Source: CAD feature listing. Evaluate the final solid. Frame: model axes, mm. Coordinates: 2 decimals unless noted, no trailing zeros. Order: outer loops, then holes, each group sorted by start corner. A loop starts at its lowest first (then second) coordinate and runs counter-clockwise, first axis right, second up. Notation, with made-up numbers: (50, -2) - (89, -2) arc R30 cw to (89, 30) - close; hole circle Ø11 at (43, 57.25). An arc over 180 degrees is marked (long way). One line per question, with ' | ' between items. Start each with the question number.
(1) Contact query for flat-ended pins moving along their axis: P1, Ø8, axis at x = -2.5, y = -0.5, coming from the +Z side; P2, Ø1.9, axis at x = 0, z = -163, coming from the -Y side; P3, Ø4, axis at x = 0, z = -163, coming from the +Y side. Output: stop coordinate, or through.
(2) Line query: line 1 along Z through (x, y) = (0, 8.9); line 2 along Y through (x, z) = (1.25, -27.5); line 3 along Z through (x, y) = (5.5, 7). Output: solid intervals per line, ascending.
(3) Section A-A (z = -77.5). Return the cut outline in (x, y).
(4) Section B-B (y = 0). Return the cut outline in (x, z), then the cut area to 3 significant figures.
(5) Section C-C (z = -163). Return the cut outline in (x, y).
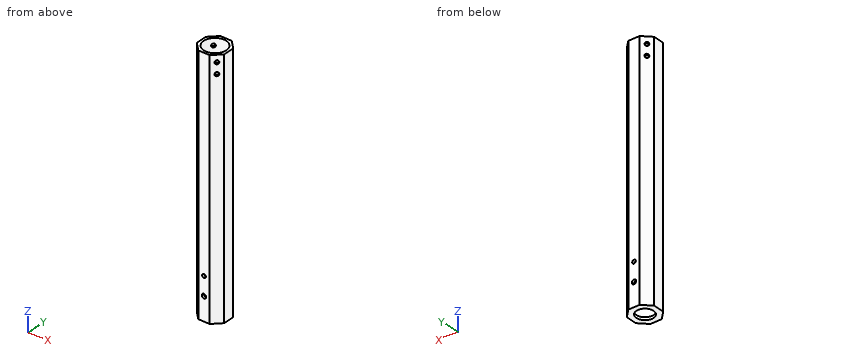
from build123d import *

# Parameters (mm, degrees)
SKETCH1_R               = 8.25
BOSS_EXTRUDE1_DEPTH     = 178
BOSS_EXTRUDE2_DEPTH     = 2
CUT_EXTRUDE1_DEPTH      = 181.554700853
CUT_EXTRUDE1_DEPTH_BACK = 181.554700853
SKETCH4_R               = 1.35
SKETCH4_R_2             = 1.6
SKETCH6_R               = 1.4
CUT_EXTRUDE2_DEPTH      = 182.611791236
CIRPATTERN1_COUNT       = 2
CIRPATTERN1_ANGLE       = 270
SKETCH7_R               = 6.269832862
CUT_EXTRUDE3_DEPTH      = 181.554700958


with BuildPart() as part:
    # Sketch1 → Boss-Extrude1 (new body)
    with BuildSketch(Plane.XY):
        Polygon((10, 4.142135624), (4.142135624, 10), (-4.142135624, 10), (-10, 4.142135624), (-10, -4.142135624), (-4.142135624, -10), (4.142135624, -10), (10, -4.142135624), align=None)
        Circle(SKETCH1_R, mode=Mode.SUBTRACT)
    extrude(amount=-BOSS_EXTRUDE1_DEPTH)

    # Sketch2 → Boss-Extrude2 (add)
    with BuildSketch(Plane(origin=(0, 0, -178), x_dir=(-1, 0, 0), z_dir=(0, 0, -1))):
        Polygon((-10, 4.142135624), (-10, -4.142135624), (-4.142135624, -10), (4.142135624, -10), (10, -4.142135624), (10, 4.142135624), (4.142135624, 10), (-4.142135624, 10), align=None)
    extrude(amount=BOSS_EXTRUDE2_DEPTH)

    # Sketch4 → Cut-Extrude1 (cut, two sides: drawn at the far end of the back side and taken through both)
    with BuildSketch(Plane(origin=(0, 0, 0), x_dir=(1, 0, 0), z_dir=(0, 1, 0)).offset(-CUT_EXTRUDE1_DEPTH_BACK)):
        with Locations(Location((0, 149.5, 0), (0, 0, 270))):
            Circle(SKETCH4_R)
        with Locations(Location((0, 163, 0), (0, 0, 270))):
            Circle(SKETCH4_R_2)
    extrude(amount=CUT_EXTRUDE1_DEPTH + CUT_EXTRUDE1_DEPTH_BACK, mode=Mode.SUBTRACT)

    # Sketch6 → Cut-Extrude2 (cut, through all)
    with BuildSketch(Plane(origin=(-7.071067812, 7.071067812, 0), x_dir=(0, 0, 1), z_dir=(-0.7071067811865476, 0.7071067811865476, 0))):
        with Locations(Location((-13, 0, 0), (0, 0, 270))):
            Circle(SKETCH6_R)
        with Locations(Location((-5, 0, 0), (0, 0, 270))):
            Circle(SKETCH6_R)
    cut_extrude2 = extrude(amount=-CUT_EXTRUDE2_DEPTH, mode=Mode.SUBTRACT)

    # CirPattern1: Cut-Extrude2 ×2 about axis
    cirpattern1_axis = Axis((0, 0, 6.85), (0, 0, -1))
    for i in range(1, CIRPATTERN1_COUNT):
        add(cut_extrude2.rotate(cirpattern1_axis, i * CIRPATTERN1_ANGLE / (CIRPATTERN1_COUNT - 1)), mode=Mode.SUBTRACT)

    # Sketch7 → Cut-Extrude3 (cut, through all)
    with BuildSketch(Plane(origin=(0, 0, -180), x_dir=(-1, 0, 0), z_dir=(0, 0, -1))):
        Circle(SKETCH7_R)
    extrude(amount=-CUT_EXTRUDE3_DEPTH, mode=Mode.SUBTRACT)


solid = part.part
Response values:
1) P1: stops at z = -178 | P2: passes through | P3: stops at y = 10
2) line 1: z = -180 to -164.6, -161.4 to -150.85, -148.15 to 0 | line 2: y = -10 to -8.15, 8.15 to 10 | line 3: z = -180 to -13.91, -12.09 to -5.91, -4.09 to 0
3) outline: (-10, -4.14) - (-4.14, -10) - (4.14, -10) - (10, -4.14) - (10, 4.14) - (4.14, 10) - (-4.14, 10) - (-10, 4.14) - close; hole circle Ø16.5 at (0, 0)
4) outline: (-10, -180) - (-6.27, -180) - (-6.27, -178) - (-8.25, -178) - (-8.25, 0) - (-10, 0) - close; (6.27, -180) - (10, -180) - (10, 0) - (8.25, 0) - (8.25, -178) - (6.27, -178) - close | area: 638 mm²
5) outline: (-10, -4.14) - (-4.14, -10) - (-1.6, -10) - (-1.6, -8.09) arc R8.25 cw to (-1.6, 8.09) - (-1.6, 10) - (-4.14, 10) - (-10, 4.14) - close; (1.6, -10) - (4.14, -10) - (10, -4.14) - (10, 4.14) - (4.14, 10) - (1.6, 10) - (1.6, 8.09) arc R8.25 cw to (1.6, -8.09) - close
